The model under review builds one solid part; all positions refer to its coordinate system, in mm. Face numbers are marked on the shaded views. A direction names the side the tool comes from. Round coordinates to 2 decimals unless told otherwise and drop trailing zeros. Order: outer loops, then holes, each group sorted by start corner. A loop starts at its lowest first (then second) coordinate and runs counter-clockwise, first axis right, second up.
from build123d import *

# Parameters (mm, degrees)
LEG_START          = -45
SKETCH1_W          = 12
SKETCH1_H          = 12
LEG_DEPTH          = 45
FOOT_PAD_START     = -45
SKETCH2_W          = 12
SKETCH2_H          = 18
FOOT_PAD_DEPTH     = 5
FOOT_HOLE_M4_START = -45.5
SKETCH3_R          = 2.25
FOOT_HOLE_M4_DEPTH = 6


with BuildPart() as part:
    # Sketch1 → Leg (new body)
    with BuildSketch(Plane(origin=(0, 0, 0), x_dir=(1, 0, 0), z_dir=(0, 1, 0)).offset(LEG_START)):
        Rectangle(SKETCH1_W, SKETCH1_H)
    extrude(amount=LEG_DEPTH)

    # Sketch2 → Foot_Pad (add)
    with BuildSketch(Plane(origin=(0, 0, 0), x_dir=(1, 0, 0), z_dir=(0, 1, 0)).offset(FOOT_PAD_START)):
        with Locations((0, -9)):
            Rectangle(SKETCH2_W, SKETCH2_H)
    extrude(amount=FOOT_PAD_DEPTH)

    # Sketch3 → Foot_Hole_M4 (cut)
    with BuildSketch(Plane(origin=(0, 0, 0), x_dir=(1, 0, 0), z_dir=(0, 1, 0)).offset(FOOT_HOLE_M4_START)):
        with Locations(Location((0, -13, 0), (0, 0, 270))):
            Circle(SKETCH3_R)
    extrude(amount=FOOT_HOLE_M4_DEPTH, mode=Mode.SUBTRACT)


solid = part.part
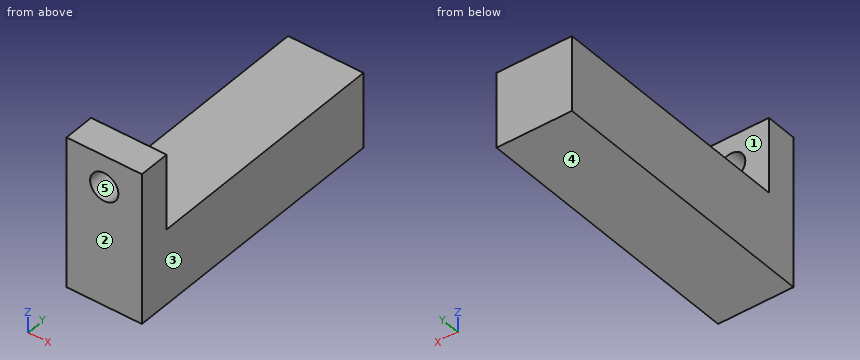
(1) The part is to be moulded in two halves that separate along X. For the marked faces 3, 4 and 5, say which applies: pulls with the +X half, pulls with the -X half, needs draft (parallel to the pull), parting line crosses it, or undercut.
(2) We need section C-C (x = -4.25). Give the boundary of the cut face in (y, z).
(3) We need section B-B (z = 13). Give the boundary of the cut face in (x, y), and give its area (3 significant figures).
(4) Tool access review of the marked faces 1 and 2: name each direction out of +Z, -Z, +X, -X, +Y, -Y from which nothing blocks a thin tool from reaching the whole face with its end or side.
(5) We need section A-A (x = 0). Give the boundary of the cut face in (y, z).
(6) Clearance check with flat-ended pins moving along their axes: P1, Ø6, axis at x = -1, y = -21.5, coming from the +Z side; P2, Ø5, axis at x = 0, z = 13, coming from the +Y side. State where each tip first meets the part, or that it passes through.
(7) We need section D-D (y = -37). Give the boundary of the cut face in (x, z), and give its area (3 significant figures).
(8) To check wall thickness, follow L1, parallel to X at y = -43.1, z = 13; L2, parallel to Z at x = 0, y = -42.3; L3, parallel to Y at x = 3.5, z = 11.5. State the ranges of each line that lie inside material, in increasing order.
Verdict:
1. face 3: pulls with the +X half
1. face 4: needs draft
1. face 5: undercut
2. outline: (-45, -6) - (0, -6) - (0, 6) - (-40, 6) - (-40, 18) - (-45, 18) - close
3. outline: (-6, -45) - (-2.25, -45) - (-2.25, -40) - (-6, -40) - close; (2.25, -45) - (6, -45) - (6, -40) - (2.25, -40) - close
3. area: 37.5 mm2
4. face 1: +Z, +X, -X, +Y
4. face 2: +Z, -Z, +X, -X, -Y
5. outline: (-45, -6) - (0, -6) - (0, 6) - (-40, 6) - (-40, 10.75) - (-45, 10.75) - close; (-45, 15.25) - (-40, 15.25) - (-40, 18) - (-45, 18) - close
6. P1: stops at z = 6
6. P2: stops at y = -40
7. outline: (-6, -6) - (6, -6) - (6, 6) - (-6, 6) - close
7. area: 144 mm2
8. L1: x = -6 to -2.25, 2.25 to 6
8. L2: z = -6 to 10.75, 15.25 to 18
8. L3: y = -45 to -40
